from build123d import *

# Parameters (mm, degrees)
ESQUISSE1_W                  = 80
ESQUISSE1_H                  = 182
BOSS_EXTRU_1_DEPTH           = 20
ENL_V_MAT_EXTRU_1_DEPTH      = 200.809909664
ENL_V_MAT_EXTRU_1_DEPTH_BACK = 200.809909664
ESQUISSE2_R                  = 11
CHANFREIN1_SIZE              = 20
ESQUISSE3_R                  = 21
ENL_V_MAT_EXTRU_2_DEPTH      = 12.5
ESQUISSE4_R                  = 15
ENL_V_MAT_EXTRU_3_DEPTH      = 2
ENL_V_MAT_EXTRU_4_DEPTH      = 200.809909664
ENL_V_MAT_EXTRU_4_DEPTH_BACK = 200.809909664
ESQUISSE5_W                  = 10
ESQUISSE5_H                  = 20


with BuildPart() as part:
    # Esquisse1 → Boss.-Extru.1 (new body)
    with BuildSketch(Plane.XY):
        with Locations((40, 91)):
            Rectangle(ESQUISSE1_W, ESQUISSE1_H)
    extrude(amount=BOSS_EXTRU_1_DEPTH)

    # Esquisse2 → Enlèv. mat.-Extru.1 (cut, two sides: drawn at the far end of the back side and taken through both)
    with BuildSketch(Plane.XY.offset(20).offset(-ENL_V_MAT_EXTRU_1_DEPTH_BACK)):
        with Locations((40, 155)):
            Circle(ESQUISSE2_R)
    extrude(amount=ENL_V_MAT_EXTRU_1_DEPTH + ENL_V_MAT_EXTRU_1_DEPTH_BACK, mode=Mode.SUBTRACT)

    # Chanfrein1
    chanfrein1_edges = [part.edges().sort_by_distance(p)[0] for p in [
        (0, 182, 10),
        (80, 182, 10),
    ]]
    chamfer(chanfrein1_edges, length=CHANFREIN1_SIZE)

    # Esquisse3 → Enlèv. mat.-Extru.2 (cut)
    with BuildSketch(Plane.XY.offset(20)):
        with Locations((40, 155)):
            Circle(ESQUISSE3_R)
    extrude(amount=-ENL_V_MAT_EXTRU_2_DEPTH, mode=Mode.SUBTRACT)

    # Esquisse4 → Enlèv. mat.-Extru.3 (cut)
    with BuildSketch(Plane.XY.offset(7.5)):
        with Locations((40, 155)):
            Circle(ESQUISSE4_R)
    extrude(amount=-ENL_V_MAT_EXTRU_3_DEPTH, mode=Mode.SUBTRACT)

    # Esquisse5 → Enlèv. mat.-Extru.4 (cut, two sides: drawn at the far end of the back side and taken through both)
    with BuildSketch(Plane.XY.offset(20).offset(-ENL_V_MAT_EXTRU_4_DEPTH_BACK)):
        with Locations((75, 30)):
            Rectangle(ESQUISSE5_W, ESQUISSE5_H)
        with Locations((5, 30)):
            Rectangle(ESQUISSE5_W, ESQUISSE5_H)
    extrude(amount=ENL_V_MAT_EXTRU_4_DEPTH + ENL_V_MAT_EXTRU_4_DEPTH_BACK, mode=Mode.SUBTRACT)


solid = part.part
Input: part model. Units: mm. Frame: model coordinates. A direction names the side the tool comes from. Round coordinates to 2 decimals unless told otherwise and drop trailing zeros. Order: outer loops, then holes, each group sorted by start corner. A loop starts at its lowest first (then second) coordinate and runs counter-clockwise, first axis right, second up. Notation, with made-up numbers: (40, -10.75) - (93, -10.75) arc R22 ccw to (93, -0.75) - close; hole circle Ø2 at (0.5, 10.5). An arc over 180 degrees is marked (long way). Use a Markdown table: item, result.
1. Access query for faces 1 (the face through (5, 40, 10)), 2 (the face through (10, 172, 10)), 3 (the face through (37.27, 175.82, 13.84)), 4 (the face through (70, 30, 10)). Directions: +Z, -Z, +X, -X, +Y, -Y. A direction counts if a zero-diameter tool reaches every point of the face in a straight line with its end or side. Return the directions, or none.
Evaluation:
| item | result |
|---|---|
| face 1 | +Z, -Z, -X |
| face 2 | +Z, -Z, -X, +Y |
| face 3 | +Z |
| face 4 | +Z, -Z, +X |
2. Mould query, pull axis X, two halves, no side actions, for faces 5 (the face through (80, 10, 10)), 6 (the face through (75, 40, 10)), 7 (the face through (36.748, 140.357, 6.514)). Classes: +X half, -X half, draft (parallel to the pull), parting line (faces both ways), or undercut.
Evaluation:
| item | result |
|---|---|
| face 5 | +X half |
| face 6 | draft |
| face 7 | undercut |
3. Material intervals for probe 1 along X at (y, z) = (155, 3.3); probe 2 along Y at (x, z) = (40, 13.25); probe 3 along Y at (x, z) = (40, 3.2), sorted ascending.
Evaluation:
| item | result |
|---|---|
| probe 1 | 0 to 29, 51 to 80 |
| probe 2 | 0 to 134, 176 to 182 |
| probe 3 | 0 to 144, 166 to 182 |
4. First-contact query: pin 1 (1.5 mm diameter, centred on y = 27.5, z = 14.5, fed in from -X); pin 2 (6 mm diameter, centred on x = 9, z = 14, fed in from +Y); pin 3 (8 mm diameter, centred on x = 14.5, y = 37.5, fed in from -Z); pin 4 (9 mm diameter, centred on x = 32.5, y = 161.5, fed in from +Z). Flat tips, straight axial feed; report the tip coordinate or a pass-through.
Evaluation:
| item | result |
|---|---|
| pin 1 | x = 10 |
| pin 2 | y = 174 |
| pin 3 | z = 0 |
| pin 4 | z = 5.5 |
5. Section C-C on y = 155. Return the cut outline in (x, z).
Evaluation:
| item | result |
|---|---|
| outline | (0, 0) - (29, 0) - (29, 5.5) - (25, 5.5) - (25, 7.5) - (19, 7.5) - (19, 20) - (0, 20) - close; (51, 0) - (80, 0) - (80, 20) - (61, 20) - (61, 7.5) - (55, 7.5) - (55, 5.5) - (51, 5.5) - close |
6. Section A-A on x = 40. Return the cut outline in (y, z), then the cut area to 3 significant figures.
Evaluation:
| item | result |
|---|---|
| outline | (0, 0) - (144, 0) - (144, 5.5) - (140, 5.5) - (140, 7.5) - (134, 7.5) - (134, 20) - (0, 20) - close; (166, 0) - (182, 0) - (182, 20) - (176, 20) - (176, 7.5) - (170, 7.5) - (170, 5.5) - (166, 5.5) - close |
| area | 2,930 mm^2 |
7. Section B-B on z = 16.25. Return the cut outline in (x, y), then the cut area to 3 significant figures.
Evaluation:
| item | result |
|---|---|
| outline | (0, 0) - (80, 0) - (80, 20) - (70, 20) - (70, 40) - (80, 40) - (80, 162) - (60, 182) - (20, 182) - (0, 162) - (0, 40) - (10, 40) - (10, 20) - (0, 20) - close; hole circle Ø42 at (40, 155) |
| area | 12,400 mm^2 |
